```python
from build123d import *

# Parameters (mm, degrees)
SKETCH1_R               = 1.5
BOSS_EXTRUDE1_DEPTH     = 3.175
CUT_EXTRUDE1_DEPTH      = 131.960225355
CUT_EXTRUDE1_DEPTH_BACK = 131.960225355
CUT_EXTRUDE2_DEPTH      = 131.960225355
CUT_EXTRUDE2_DEPTH_BACK = 131.960225355
CUT_EXTRUDE3_DEPTH      = 131.960225355
CUT_EXTRUDE3_DEPTH_BACK = 131.960225355
SKETCH4_R               = 1.6
CUT_EXTRUDE4_DEPTH      = 40


with BuildPart() as part:
    # Sketch1 → Boss-Extrude1 (new body)
    with BuildSketch(Plane(origin=(0, 0, 0), x_dir=(1, 0, 0), z_dir=(0, 1, 0))):
        with BuildLine():
            Line((-10.5, 0), (-10.5, -120))
            ThreePointArc((-10.5, -120), (0, -130.5), (10.5, -120))
            Line((10.5, -120), (10.5, 0))
            ThreePointArc((10.5, 0), (0, 10.5), (-10.5, 0))
        make_face()
        with Locations(Location((0, 0, 0), (0, 0, 270))):
            Circle(SKETCH1_R, mode=Mode.SUBTRACT)
        with Locations(Location((0, -120, 0), (0, 0, 270))):
            Circle(SKETCH1_R, mode=Mode.SUBTRACT)
    extrude(amount=BOSS_EXTRUDE1_DEPTH)

    # Sketch2 → Cut-Extrude1 (cut, two sides: drawn at the far end of the back side and taken through both)
    with BuildSketch(Plane.XZ.offset(-CUT_EXTRUDE1_DEPTH_BACK)):
        with BuildLine():
            ThreePointArc((0, 18.75), (1.25, 20), (0, 21.25))
            ThreePointArc((0, 21.25), (-1.25, 20), (0, 18.75))
        make_face()
        with BuildLine():
            ThreePointArc((0, 25.25), (-1.25, 24), (0, 22.75))
            ThreePointArc((0, 22.75), (1.25, 24), (0, 25.25))
        make_face()
    extrude(amount=CUT_EXTRUDE1_DEPTH + CUT_EXTRUDE1_DEPTH_BACK, mode=Mode.SUBTRACT)

    # Sketch3 → Cut-Extrude2 (cut, two sides: drawn at the far end of the back side and taken through both)
    with BuildSketch(Plane(origin=(0, 3.175, 0), x_dir=(1, 0, 0), z_dir=(0, 1, 0)).offset(-CUT_EXTRUDE2_DEPTH_BACK)):
        with BuildLine():
            ThreePointArc((0, -97.25), (1.25, -96), (0, -94.75))
            ThreePointArc((0, -94.75), (-1.25, -96), (0, -97.25))
        make_face()
        with BuildLine():
            ThreePointArc((0, -98.75), (-1.25, -100), (0, -101.25))
            ThreePointArc((0, -101.25), (1.25, -100), (0, -98.75))
        make_face()
    extrude(amount=CUT_EXTRUDE2_DEPTH + CUT_EXTRUDE2_DEPTH_BACK, mode=Mode.SUBTRACT)

    # Sketch4 → Cut-Extrude3 (cut, two sides: drawn at the far end of the back side and taken through both)
    with BuildSketch(Plane(origin=(0, 3.175, 0), x_dir=(1, 0, 0), z_dir=(0, 1, 0)).offset(-CUT_EXTRUDE3_DEPTH_BACK)):
        with Locations(Location((0, -35.15, 0), (0, 0, 270))):
            Circle(SKETCH4_R)
        with Locations(Location((0, -85.15, 0), (0, 0, 270))):
            Circle(SKETCH4_R)
    extrude(amount=CUT_EXTRUDE3_DEPTH + CUT_EXTRUDE3_DEPTH_BACK, mode=Mode.SUBTRACT)

    # Sketch5 → Cut-Extrude4 (cut)
    with BuildSketch(Plane.XZ):
        with BuildLine():
            Line((-8.5, 10), (-8.5, 50))
            ThreePointArc((-8.5, 50), (-7.5, 51), (-6.5, 50))
            Line((-6.5, 50), (-6.5, 10))
            ThreePointArc((-6.5, 10), (-7.5, 9), (-8.5, 10))
        make_face()
        with BuildLine():
            Line((6.5, 50), (6.5, 10))
            ThreePointArc((6.5, 10), (7.5, 9), (8.5, 10))
            Line((8.5, 10), (8.5, 50))
            ThreePointArc((8.5, 50), (7.5, 51), (6.5, 50))
        make_face()
        with BuildLine():
            Line((8.5, 110), (8.5, 70))
            ThreePointArc((8.5, 70), (7.5, 69), (6.5, 70))
            Line((6.5, 70), (6.5, 110))
            ThreePointArc((6.5, 110), (7.5, 111), (8.5, 110))
        make_face()
        with BuildLine():
            Line((-6.5, 70), (-6.5, 110))
            ThreePointArc((-6.5, 110), (-7.5, 111), (-8.5, 110))
            Line((-8.5, 110), (-8.5, 70))
            ThreePointArc((-8.5, 70), (-7.5, 69), (-6.5, 70))
        make_face()
    extrude(amount=-CUT_EXTRUDE4_DEPTH, mode=Mode.SUBTRACT)


solid = part.part
```
Could you check a few things on this model? Use its own coordinates, in mm. A direction names the side the tool comes from. Round coordinates to 2 decimals unless told otherwise and drop trailing zeros. Write each loop counter-clockwise with the first axis right and the second up, starting at its lowest first coordinate (ties: lowest second). Pieces come first, ordered by that corner, then holes.
(1) Which directions (+Z, -Z, +X, -X, +Y, -Y) give clear straight access to the entire face, cutting with the end or side of a thin tool? Please do faces 4 (the face through (-10.5, 2, 59)), 5 (the face through (-6.5, 2, 30)).
Findings below:
face 4: +Z, -Z, -X, +Y, -Y
face 5: +Y, -Y
(2) Suppose I cut it at B-B on z = 20. Write out the boundary of the cut face in (x, y) (3 decimals).
Findings below:
outline: (-10.5, 0) - (-8.5, 0) - (-8.5, 3.175) - (-10.5, 3.175) - close; (-6.5, 0) - (-1.25, 0) - (-1.25, 3.175) - (-6.5, 3.175) - close; (1.25, 0) - (6.5, 0) - (6.5, 3.175) - (1.25, 3.175) - close; (8.5, 0) - (10.5, 0) - (10.5, 3.175) - (8.5, 3.175) - close
(3) Thinking about a two-plate mould opening in Z: for faces 1 (the face through (10.5, 2, 61)), 2 (the face through (-6.5, 2, 90)), 3 (the face through (-0.2, 1.6, 130.5)), which applies, +Z half, -Z half, draft (parallel to the pull), parting line (faces both ways), or undercut?
Findings below:
face 1: draft
face 2: undercut
face 3: +Z half
(4) Suppose I cut it at C-C on y = 1.7. State how many separate pieces and enclosed holes the cut face has, and give its area (3 significant figures).
Findings below:
separate pieces: 1
enclosed holes: 12
area: 2,480 mm2
(5) Suppose I cut it at A-A on z = 107.5. Write out the boundary of the cut face in (x, y) (3 decimals).
Findings below:
outline: (-10.5, 0) - (-8.5, 0) - (-8.5, 3.175) - (-10.5, 3.175) - close; (-6.5, 0) - (6.5, 0) - (6.5, 3.175) - (-6.5, 3.175) - close; (8.5, 0) - (10.5, 0) - (10.5, 3.175) - (8.5, 3.175) - close
(6) If I drill on probe 1 along X at (y, z) = (1.5, 35.15); probe 2 along X at (y, z) = (2.05, 83); probe 3 along X at (y, z) = (1.6, 96), over which ranges is the centre line in solid material (lowest first)?
Findings below:
probe 1: x = -10.5 to -8.5, -6.5 to -1.6, 1.6 to 6.5, 8.5 to 10.5
probe 2: x = -10.5 to -8.5, -6.5 to 6.5, 8.5 to 10.5
probe 3: x = -10.5 to -8.5, -6.5 to -1.25, 1.25 to 6.5, 8.5 to 10.5
